Here's how the part is built. I have some questions about the finished solid (model axes, mm). Face numbers are marked on the shaded views. A direction names the side the tool comes from. Coordinates: 2 decimals unless noted, no trailing zeros. Order: outer loops, then holes, each group sorted by start corner. A loop starts at its lowest first (then second) coordinate and runs counter-clockwise, first axis right, second up.
```python
from build123d import *

# Parameters (mm, degrees)
BOSS_EXTRU_1_DEPTH      = 28
ESQUISSE3_R             = 1.625
ENL_V_MAT_EXTRU_1_DEPTH = 16
ESQUISSE4_R             = 2.125
ENL_V_MAT_EXTRU_2_DEPTH = 10


with BuildPart() as part:
    # Esquisse1 → Boss.-Extru.1 (new body)
    with BuildSketch(Plane.XY):
        Polygon((0, 0), (5, 0), (5, -11), (15, -11), (15, -16), (0, -16), align=None)
    extrude(amount=BOSS_EXTRU_1_DEPTH)

    # Esquisse3 → Enlèv. mat.-Extru.1 (cut, through all)
    with BuildSketch(Plane.ZY):
        with Locations((25.25, -2)):
            Circle(ESQUISSE3_R)
        with Locations((2.75, -14)):
            Circle(ESQUISSE3_R)
        with Locations((25.25, -14)):
            Circle(ESQUISSE3_R)
        with Locations((2.75, -2)):
            Circle(ESQUISSE3_R)
    extrude(amount=-ENL_V_MAT_EXTRU_1_DEPTH, mode=Mode.SUBTRACT)

    # Esquisse4 → Enlèv. mat.-Extru.2 (cut)
    with BuildSketch(Plane(origin=(0, -11, 0), x_dir=(1, 0, 0), z_dir=(0, 1, 0))):
        with Locations((10, -9)):
            Circle(ESQUISSE4_R)
        with Locations((10, -19)):
            Circle(ESQUISSE4_R)
    extrude(amount=-ENL_V_MAT_EXTRU_2_DEPTH, mode=Mode.SUBTRACT)


solid = part.part
```
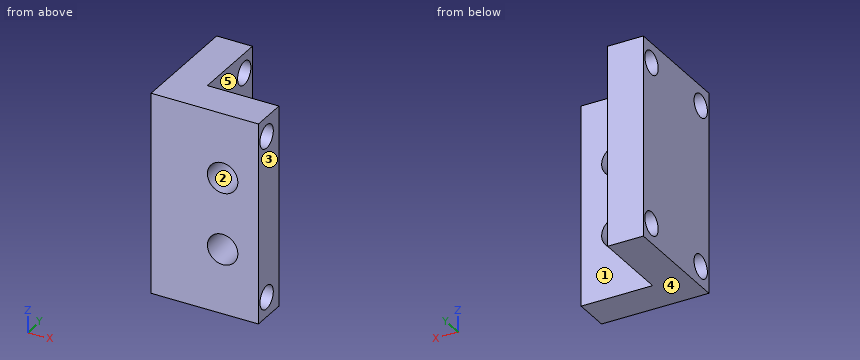
Q1. For the marked faces 4 and 5, which set-ups out of +Z, -Z, +X, -X, +Y, -Y let a thin tool reach every point of the face, with its end or its side?
Q2. If we section it at B-B on z = 2.75: Write out the boundary of the cut face in (x, y) (3 decimals), then the cut area to 3 significant figures.
Q3. If we section it at D-D on y = -11.75: Write out the boundary of the cut face in (x, z) (3 decimals), then the cut area to 3 significant figures.
Q4. We'd pull the mould along X, two halves only. Please class the marked faces 1, 2 and 3: pulls with the +X half, pulls with the -X half, needs draft (parallel to the pull), parting line crosses it, or undercut.
Q5. Will these pins go through, and if not, where does the flat tip stop? pin 1 (5 mm diameter, centred on y = -14, z = 25.25, fed in from -X); pin 2 (5.5 mm diameter, centred on x = 10, z = 9, fed in from +Y); pin 3 (5 mm diameter, centred on y = -2, z = 25.25, fed in from +X).
Q6. If we section it at A-A on x = 10: Write out the boundary of the cut face in (y, z) (3 decimals), then the cut area to 3 significant figures.
Q7. I need wall thicknesses on L1, parallel to Y at x = 1.5, z = 2.75 (3 decimals); L2, parallel to Z at x = 3.75, y = -12.75; L3, parallel to X at y = -12.75, z = 9 (3 decimals). Which ranges of each line are inside material? Lowest first, please.
Q8. If we section it at C-C on x = 1.75: Write out the boundary of the cut face in (y, z) (3 decimals).
Reply:
1. face 4: -Z, +X, -X, +Y, -Y
1. face 5: +Z, -Z, +X, +Y
2. outline: (0, -16) - (15, -16) - (15, -15.625) - (0, -15.625) - close; (0, -12.375) - (15, -12.375) - (15, -11) - (5, -11) - (5, -3.625) - (0, -3.625) - close; (0, -0.375) - (5, -0.375) - (5, 0) - (0, 0) - close
2. area: 65.0 mm2
3. outline: (0, 0) - (15, 0) - (15, 28) - (0, 28) - close; hole circle Ø4.25 at (10, 9); hole circle Ø4.25 at (10, 19)
3. area: 392 mm2
4. face 1: needs draft
4. face 2: undercut
4. face 3: pulls with the +X half
5. pin 1: stops at x = 0
5. pin 2: stops at y = -11
5. pin 3: stops at x = 5
6. outline: (-16, 0) - (-11, 0) - (-11, 6.875) - (-16, 6.875) - close; (-16, 11.125) - (-11, 11.125) - (-11, 16.875) - (-16, 16.875) - close; (-16, 21.125) - (-11, 21.125) - (-11, 28) - (-16, 28) - close; hole circle Ø3.25 at (-14, 2.75); hole circle Ø3.25 at (-14, 25.25)
6. area: 80.9 mm2
7. L1: y = -16 to -15.625, -12.375 to -3.625, -0.375 to 0
7. L2: z = 0 to 1.71, 3.79 to 24.21, 26.29 to 28
7. L3: x = 0 to 7.875, 12.125 to 15
8. outline: (-16, 0) - (0, 0) - (0, 28) - (-16, 28) - close; hole circle Ø3.25 at (-14, 2.75); hole circle Ø3.25 at (-14, 25.25); hole circle Ø3.25 at (-2, 2.75); hole circle Ø3.25 at (-2, 25.25)
